```python
from build123d import *

# Parameters (mm, degrees)
F1_DEPTH = 57
F2_R     = 10
F3_R     = 8
F4_R     = 19.5
F5_DEPTH = 23.0736274766


with BuildPart() as f1:
    # F0 (on Front) → F1 (new body, symmetric)
    with BuildSketch(Plane.XZ):
        with BuildLine():
            ThreePointArc((76.3113958567, 97.9800145677), (65.3139848131, 170.5380837413), (0, 204))
            ThreePointArc((0, 204), (-65.3139848131, 170.5380837413), (-76.3113958567, 97.9800145677))
            ThreePointArc((-76.3113958567, 97.9800145677), (-64.5868234444, 82.0664049994), (-45.774399408, 76))
            Line((-45.774399408, 76), (-36.437930815, 76))
            ThreePointArc((-36.437930815, 76), (-46.804780385, 36.5859685512), (-43.1011872895, -4))
            Line((-43.1011872895, -4), (43.1011872895, -4))
            ThreePointArc((43.1011872895, -4), (46.804780385, 36.5859685512), (36.437930815, 76))
            Line((36.437930815, 76), (45.774399408, 76))
            ThreePointArc((45.774399408, 76), (64.5868234444, 82.0664049994), (76.3113958567, 97.9800145677))
        make_face()
        with BuildLine():
            ThreePointArc((-28.4035311639, 15), (-27.8807773056, 46.3973285977), (-17.4047398621, 76))
            Line((-17.4047398621, 76), (17.4047398621, 76))
            ThreePointArc((17.4047398621, 76), (27.8807773056, 46.3973285977), (28.4035311639, 15))
            Line((28.4035311639, 15), (-28.4035311639, 15))
        make_face(mode=Mode.SUBTRACT)
        with BuildLine():
            ThreePointArc((-45.774399408, 95), (-53.4872363848, 97.4871432148), (-58.2941509783, 104.0115058422))
            ThreePointArc((-58.2941509783, 104.0115058422), (-49.8932465977, 159.4384966818), (0, 185))
            ThreePointArc((0, 185), (49.8932465977, 159.4384966818), (58.2941509783, 104.0115058422))
            ThreePointArc((58.2941509783, 104.0115058422), (53.4872363848, 97.4871432148), (45.774399408, 95))
            Line((45.774399408, 95), (-45.774399408, 95))
        make_face(mode=Mode.SUBTRACT)
    extrude(amount=F1_DEPTH, both=True)

    # F2
    f2_edges = [f1.edges().sort_by_distance(p)[0] for p in [
        (-43.101187, 0, -4),
        (43.101187, 0, -4),
    ]]
    fillet(f2_edges, radius=F2_R)

    # F3
    f3_edges = [f1.edges().sort_by_distance(p)[0] for p in [
        (-17.40474, 0, 76),
        (17.40474, 0, 76),
        (28.403531, 0, 15),
        (35.177601, 0, -4),
        (-28.403531, 0, 15),
    ]]
    fillet(f3_edges, radius=F3_R)

    # F4 (on face) → F5 (cut, through all)
    with BuildSketch(Plane.XY.offset(95)):
        Circle(F4_R)
    extrude(amount=-F5_DEPTH, mode=Mode.SUBTRACT)


solid = f1.part
```
Model file for the job. Use its own axes, mm. A direction names the side the tool comes from. Round coordinates to 2 decimals unless told otherwise and drop trailing zeros. Loops run counter-clockwise (first coordinate to the right, second up) from the corner with the lowest first, then second, coordinate; pieces in that order, holes last. Notation, with made-up numbers: M 15.5,62 L 40.5,62 A21 ccw 40.5,101 Z; hole C 55,22 d2. An arc over 180 degrees is marked long. Put each result on its own line as item: value. Start each with the question number.
Item 1: Cut at A-A (x = 0). List the corners of the cut face in (y, z).
Item 2: Cut at C-C (y = 0). List the corners of the cut face in (x, z), then the cut area to 3 significant figures.
Item 3: Mould opens along Z. For faces 5 (the face through (0, -57, 93)), 6 (the face through (-16.84, -13.46, 74.74)), 7 (the face through (27.59, -0.8, 47.93)), 8 (the face through (0, -1, -4)) say: released by +Z, released by -Z, zero draft, split by the parting line, or undercut.
Item 4: Drill centre lines: line 1 along Z through (x, y) = (3.5, -39); line 2 along Z through (x, y) = (-15.5, 40); line 3 along Y through (x, z) = (0, 89). Where is each one in solid material? Low to high.
Item 5: Cut at B-B (y = -23.5). List the corners of the cut face in (x, z).
Item 6: Drop flat-ended pins along their axis: P1, Ø5, axis at y = 44.5, z = 158.5, coming from the -X side; P2, Ø4, axis at y = -14, z = 50.5, coming from the +X side; P3, Ø8, axis at x = -15.5, y = -15, coming from the +Z side. Give the stop position or say it passes through.
Item 7: Cut at D-D (x = 54.5). List the corners of the cut face in (y, z), then the cut area to 3 significant figures.
Item 8: 3-axis set-ups, long thin cutter, end or side, ignore diameter. For faces 1 (the face through (21, -1, 95)), 2 (the face through (-41, -1, 76)), 3 (the face through (41, -1, 76)), 4 (the face through (-14.37, 13.18, 86.19)): which of +Z, -Z, +X, -X, +Y, -Y reach the whole face in a straight line?
Answer block:
1. outline: M -57,-4 L 57,-4 L 57,15 L -57,15 Z; M -57,76 L -19.5,76 L -19.5,95 L -57,95 Z; M -57,185 L 57,185 L 57,204 L -57,204 Z; M 19.5,76 L 57,76 L 57,95 L 19.5,95 Z
2. outline: M -76.31,97.98 A32.2 ccw -45.77,76 L -36.44,76 A117.64 ccw -44.99,4.07 A10 ccw -35.18,-4 L 35.18,-4 A10 ccw 44.99,4.07 A117.64 ccw 36.44,76 L 45.77,76 A32.2 ccw 76.31,97.98 A80.47 ccw long Z; hole M -58.29,104.01 A13.2 ccw -45.77,95 L -19.5,95 L -19.5,71.93 A8 ccw -19.74,71.48 A97.5 ccw -29.2,22.46 A8 ccw -21.22,15 L 21.22,15 A8 ccw 29.2,22.46 A97.5 ccw 19.74,71.48 A8 ccw 19.5,71.93 L 19.5,95 L 45.77,95 A13.2 ccw 58.29,104.01 A61.47 ccw long Z
2. area: 11,100 mm2
3. face 5: zero draft
3. face 6: undercut
3. face 7: undercut
3. face 8: released by -Z
4. line 1: -4 to 15, 76 to 95, 184.9 to 203.92
4. line 2: -4 to 15, 75.43 to 95, 183.01 to 202.49
4. line 3: -57 to -19.5, 19.5 to 57
5. outline: M -76.31,97.98 A32.2 ccw -45.77,76 L -36.44,76 A117.64 ccw -44.99,4.07 A10 ccw -35.18,-4 L 35.18,-4 A10 ccw 44.99,4.07 A117.64 ccw 36.44,76 L 45.77,76 A32.2 ccw 76.31,97.98 A80.47 ccw long Z; hole M -58.29,104.01 A13.2 ccw -45.77,95 L 45.77,95 A13.2 ccw 58.29,104.01 A61.47 ccw long Z; hole M -29.2,22.46 A8 ccw -21.22,15 L 21.22,15 A8 ccw 29.2,22.46 A97.5 ccw 19.74,71.48 A8 ccw 12.53,76 L -12.53,76 A8 ccw -19.74,71.48 A97.5 ccw Z
6. P1: x = -73.63
6. P2: x = 45.2
6. P3: z = 203.17
7. outline: M -57,77.2 L 57,77.2 L 57,98.29 L -57,98.29 Z; M -57,151.97 L 57,151.97 L 57,182.74 L -57,182.74 Z
7. area: 5,910 mm2
8. face 1: +Y, -Y
8. face 2: -X, +Y, -Y
8. face 3: +X, +Y, -Y
8. face 4: none
